Part model, mm, in its own coordinate system. A direction names the side the tool comes from. Coordinates: 2 decimals unless noted, no trailing zeros. Write each loop counter-clockwise with the first axis right and the second up, starting at its lowest first coordinate (ties: lowest second). Pieces come first, ordered by that corner, then holes. Notation, with made-up numbers: (46, 28.25) -> (61, 28.25) arc R22 ccw to (61, 50.25) -> close; hole circle Ø7 at (36, -7.5). An arc over 180 degrees is marked (long way). One line per question, with ' | ' between items. Start each with the question number.
Item 1: Saw through at A-A (y = 21). List the corners of the cut face in (x, z), and give its area (3 significant figures).
Item 2: Pin check, flat tips, straight feed: pin 1 (1.5 mm diameter, centred on y = 30, z = 0.5, fed in from +X); pin 2 (1 mm diameter, centred on x = 29.5, y = 23, fed in from -Z); pin 3 (10 mm diameter, centred on y = -49.5, z = 2, fed in from -X). Stop position of each tip, or through.
Item 3: Two-plate mould, pull along X, no slides. Class faces 3 (the flat face through (-23.3, -36.5, -12.1)), 4 (the cylindrical face through (-13.77, 61.99, 7.39)): pulls with the +X half, pulls with the -X half, needs draft (parallel to the pull), parting line crosses it, or undercut.
Item 4: Saw through at B-B (z = 4). List the corners of the cut face in (x, y), and give its area (3 significant figures).
Item 5: 3-axis set-ups, long thin cutter, end or side, ignore diameter. For faces 1 (the flat face through (0, 0, 6.5)), 2 (the flat face through (0, 0, -6.5)): which of +Z, -Z, +X, -X, +Y, -Y reach the whole face in a straight line?
Item 6: Probe probe 1 along Y at (x, z) = (0, -7.8); probe 2 along Y at (x, z) = (0, 9.25). List the from-to ranges inside material, lowest first. Write a range as [from, to].
from build123d import *


with BuildPart() as f1:
    # F0 (on Front) → F1 (revolve)
    with BuildSketch(Plane.XZ):
        Polygon((0, 6.5), (0, 0), (65, 0), (65, 8.3), (63.5, 8.3), (63.5, 6.5), (44.5, 6.5), (44.5, 12.1), (43, 12.1), (43, 6.480602), (19, 6.480602), (19, 14.380602), (17.5, 14.4), (17.5, 6.5), align=None)
    revolve(axis=Axis((0, 0, 3.25), (0, 0, -1)))

    # F2: F1 across plane


with BuildPart() as f1_1:
    add(f1.part)
    add(f1.part.mirror(Plane.XY))


solid = f1_1.part
From the geometry:
1) outline: (-61.51, -8.3) -> (-59.93, -8.3) -> (-59.93, -6.5) -> (-39.23, -6.5) -> (-39.23, -12.1) -> (-37.52, -12.1) -> (-37.52, -6.48) -> (37.52, -6.48) -> (37.52, -12.1) -> (39.23, -12.1) -> (39.23, -6.5) -> (59.93, -6.5) -> (59.93, -8.3) -> (61.51, -8.3) -> (61.51, 8.3) -> (59.93, 8.3) -> (59.93, 6.5) -> (39.23, 6.5) -> (39.23, 12.1) -> (37.52, 12.1) -> (37.52, 6.48) -> (-37.52, 6.48) -> (-37.52, 12.1) -> (-39.23, 12.1) -> (-39.23, 6.5) -> (-59.93, 6.5) -> (-59.93, 8.3) -> (-61.51, 8.3) -> close | area: 1,650 mm2
2) pin 1: x = 58.05 | pin 2: z = -6.48 | pin 3: x = -47.38
3) face 3: needs draft | face 4: undercut
4) outline: circle Ø130 at (0, 0) | area: 13,300 mm2
5) face 1: +Z | face 2: -Z
6) probe 1: [-65, -63.5], [-44.5, -43], [-19, -17.5], [17.5, 19], [43, 44.5], [63.5, 65] | probe 2: [-44.5, -43], [-19, -17.5], [17.5, 19], [43, 44.5]
